Could you check a few things on this model? Use its own coordinates, in mm. A direction names the side the tool comes from. Coordinates: 2 decimals unless noted, no trailing zeros. Order: outer loops, then holes, each group sorted by start corner. A loop starts at its lowest first (then second) coordinate and runs counter-clockwise, first axis right, second up. Notation, with made-up numbers: (86.5, 83.25) - (145.5, 83.25) arc R21 cw to (145.5, 116.25) - close; hole circle Ø1 at (22.25, 35.25). An arc over 180 degrees is marked (long way). Answer as a JSON object with one key per item and string values. Group by question number.
(1) We'd pull the mould along Y, two halves only. Please class faces 6 (the flat face through (6, 13, 25.4)), 7 (the cylindrical face through (6.663, 23.155, 5.617)), 8 (the cylindrical face through (37.376, 5.586, 12.522)): pulls with the +Y half, pulls with the -Y half, needs draft (parallel to the pull), parting line crosses it, or undercut.
(2) Imagine slicing it at B-B, the plane y = 30. Write out the boundary of the cut face in (x, z), and give its area (3 significant figures).
(3) Which directions (+Z, -Z, +X, -X, +Y, -Y) give clear straight access to the entire face, cutting with the end or side of a thin tool? Please do faces 1 (the flat face through (38.1, 2, 13)), 2 (the cylindrical face through (7.114, 7.074, 12.522)), 3 (the flat face through (2, 38.1, 13)), 4 (the flat face through (22, 9.525, 13)), 5 (the cylindrical face through (16.96, 6.66, 7.87)).
(4) Please list where these lines run through material, in increasing order: probe 1 along Y at (x, z) = (12, 5); probe 2 along X at (y, z) = (21, 12.5) (3 decimals).
(5) Imagine slicing it at A-A, the plane z = 4.25. Write out the boundary of the cut face in (x, y), and give its area (3 significant figures).
(6) Will these pins go through, and if not, where does the flat tip stop? P1, Ø10, axis at y = 33.5, z = 11, coming from the +X side; P2, Ø3, axis at y = 23.5, z = 12.5, coming from the +X side (3 decimals); P3, Ø3, axis at x = 8, y = 19, coming from the +Z side.
(7) Imagine slicing it at C-C, the plane z = 12.7. Write out the boundary of the cut face in (x, y) (3 decimals).
from build123d import *

# Parameters (mm, degrees)
BOSS_EXTRUDE1_DEPTH = 25.4
SKETCH2_R           = 7.14375
BOSS_EXTRUDE2_DEPTH = 3.175
FILLET1_R           = 2.54
SKETCH3_R           = 7.14375
BOSS_EXTRUDE3_DEPTH = 3.175
FILLET2_R           = 2.54


with BuildPart() as part:
    # Sketch1 → Boss-Extrude1 (new body)
    with BuildSketch(Plane.XY):
        with BuildLine():
            Line((0, 0), (38.1, 0))
            Line((38.1, 0), (38.1, 3.81))
            ThreePointArc((38.1, 3.81), (37.356051224, 5.606051224), (35.56, 6.35))
            Line((35.56, 6.35), (8.89, 6.35))
            ThreePointArc((8.89, 6.35), (7.093948776, 7.093948776), (6.35, 8.89))
            Line((6.35, 8.89), (6.35, 35.56))
            ThreePointArc((6.35, 35.56), (5.606051224, 37.356051224), (3.81, 38.1))
            Line((3.81, 38.1), (0, 38.1))
            Line((0, 38.1), (0, 0))
        make_face()
    extrude(amount=BOSS_EXTRUDE1_DEPTH)

    # Sketch2 → Boss-Extrude2 (add)
    with BuildSketch(Plane(origin=(0, 6.35, 0), x_dir=(1, 0, 0), z_dir=(0, 1, 0))):
        with Locations((22.225, -12.7)):
            Circle(SKETCH2_R)
    extrude(amount=BOSS_EXTRUDE2_DEPTH)

    # Fillet1
    fillet1_edges = [part.edges().sort_by_distance(p)[0] for p in [
        (15.08125, 9.525, 12.7),
    ]]
    fillet(fillet1_edges, radius=FILLET1_R)

    # Sketch3 → Boss-Extrude3 (add)
    with BuildSketch(Plane(origin=(6.35, 0, 0), x_dir=(0, 0, -1), z_dir=(1, 0, 0))):
        with Locations(Location((-12.7, 22.225, 0), (0, 0, 270))):
            Circle(SKETCH3_R)
    extrude(amount=BOSS_EXTRUDE3_DEPTH)

    # Fillet2
    fillet2_edges = [part.edges().sort_by_distance(p)[0] for p in [
        (9.525, 29.36875, 12.7),
    ]]
    fillet(fillet2_edges, radius=FILLET2_R)


solid = part.part
Result set:
{
 "1": {"face 6": "needs draft", "face 7": "undercut", "face 8": "pulls with the +Y half"},
 "2": {"outline": "(0, 0) - (6.35, 0) - (6.35, 25.4) - (0, 25.4) - close", "area": "161 mm^2"},
 "3": {"face 1": "+Z, -Z, +X, +Y, -Y", "face 2": "+Z, -Z", "face 3": "+Z, -Z, +X, -X, +Y", "face 4": "+Z, -Z, +X, +Y", "face 5": "+Y"},
 "4": {"probe 1": "y = 0 to 6.35", "probe 2": "x = 0 to 9.525"},
 "5": {"outline": "(0, 0) - (38.1, 0) - (38.1, 3.81) arc R2.54 ccw to (35.56, 6.35) - (8.89, 6.35) arc R2.54 cw to (6.35, 8.89) - (6.35, 35.56) arc R2.54 ccw to (3.81, 38.1) - (0, 38.1) - close", "area": "442 mm^2"},
 "6": {"P1": "stops at x = 8.78", "P2": "stops at x = 9.525", "P3": "stops at z = 19.57"},
 "7": {"outline": "(0, 0) - (38.1, 0) - (38.1, 3.81) arc R2.54 ccw to (35.56, 6.35) - (29.369, 6.35) - (29.369, 6.985) arc R2.54 ccw to (26.829, 9.525) - (17.621, 9.525) arc R2.54 ccw to (15.081, 6.985) - (15.081, 6.35) - (8.89, 6.35) arc R2.54 cw to (6.35, 8.89) - (6.35, 15.081) - (6.985, 15.081) arc R2.54 ccw to (9.525, 17.621) - (9.525, 26.829) arc R2.54 ccw to (6.985, 29.369) - (6.35, 29.369) - (6.35, 35.56) arc R2.54 ccw to (3.81, 38.1) - (0, 38.1) - close"}
}
